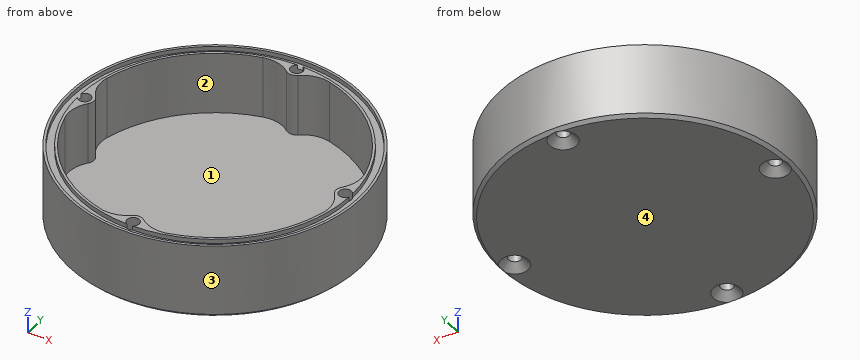
from build123d import *

# Parameters (mm, degrees)
F0_R      = 23.5
F1_DEPTH  = 12
F2_T      = -2
F3_SIZE   = 0.5
F4_R      = 1.5
F5_DEPTH  = 10
F6_R      = 5
F7_R      = 1
F8_DEPTH  = 12.001
F9_R      = 23.1
F9_R_2    = 21.9
F10_DEPTH = 0.7


# Not quite as in the source:
# - a fillet or chamfer that OpenCascade refuses, or shapes differently, is made with other operations: its cross-section is extruded or revolved along the edge and cut away or added


with BuildPart() as f1:
    # F0 (on Top) → F1 (new body)
    with BuildSketch(Plane.XY):
        Circle(F0_R)
    extrude(amount=F1_DEPTH)

    # F2
    f2_openings = [f1.faces().sort_by_distance(p)[0] for p in [
        (0, 0, 12),
    ]]
    offset(amount=F2_T, openings=f2_openings)

    # F3
    f3_edges = [f1.edges().sort_by_distance(p)[0] for p in [
        (-23.5, 0, 0),
    ]]
    chamfer(f3_edges, length=F3_SIZE)

    # F4 (on face) → F5 (join, through all)
    with BuildSketch(Plane.XY.offset(2)):
        with Locations((0, -21)):
            Circle(F4_R)
        with Locations((21, 0)):
            Circle(F4_R)
        with Locations((0, 21)):
            Circle(F4_R)
        with Locations((-21, 0)):
            Circle(F4_R)
    extrude(amount=F5_DEPTH)

    # F6
    f6_edges = [f1.edges().sort_by_distance(p)[0] for p in [
        (-21.452381, 1.430158, 7),
        (-21.452381, -1.430158, 7),
        (-1.430158, 21.452381, 7),
        (1.430158, 21.452381, 7),
        (21.452381, -1.430158, 7),
        (21.452381, 1.430158, 7),
        (-1.430158, -21.452381, 7),
        (1.430158, -21.452381, 7),
    ]]
    fillet(f6_edges, radius=F6_R)

    # F7 (on face) → F8 (cut, through all)
    with BuildSketch(Plane.XY.offset(12)):
        with Locations((0, -21)):
            Circle(F7_R)
        with Locations((21, 0)):
            Circle(F7_R)
        with Locations((0, 21)):
            Circle(F7_R)
        with Locations((-21, 0)):
            Circle(F7_R)
    extrude(amount=-F8_DEPTH, mode=Mode.SUBTRACT)

    # F9 (on face) → F10 (cut)
    with BuildSketch(Plane.XY.offset(12)):
        Circle(F9_R)
        Circle(F9_R_2, mode=Mode.SUBTRACT)
    extrude(amount=-F10_DEPTH, mode=Mode.SUBTRACT)

    # F11: chamfer of 1.2 on 4 edges, made by hand

    # F11_s1 → F11_t2 (revolve, cut)
    with BuildSketch(Plane.XZ.offset(-21)):
        Polygon((2.2, 0), (1, 1.2), (1, 0), align=None)
    revolve(axis=Axis((0, 21, 0), (0, 0, 1)), mode=Mode.SUBTRACT)

    # F11_s3 → F11_t4 (revolve, cut)
    with BuildSketch(Plane.XZ):
        Polygon((23.2, 0), (22, 1.2), (22, 0), align=None)
    revolve(axis=Axis((21, 0, 0), (0, 0, 1)), mode=Mode.SUBTRACT)

    # F11_s5 → F11_t6 (revolve, cut)
    with BuildSketch(Plane.XZ.offset(21)):
        Polygon((2.2, 0), (1, 1.2), (1, 0), align=None)
    revolve(axis=Axis((0, -21, 0), (0, 0, 1)), mode=Mode.SUBTRACT)

    # F11_s7 → F11_t8 (revolve, cut)
    with BuildSketch(Plane.XZ):
        Polygon((-18.8, 0), (-20, 1.2), (-20, 0), align=None)
    revolve(axis=Axis((-21, 0, 0), (0, 0, 1)), mode=Mode.SUBTRACT)


solid = f1.part
CAD build for the part. Positions are in the model's coordinates, mm. Face numbers are marked on the shaded views. Give positions to 0.01 mm unless a question says otherwise; leave off trailing zeros. Answer in a Markdown table with one row per item. Add a question column.
Item 1: Mould opens along Y. For the marked faces 1, 2, 3 and 4 say: +Y half, -Y half, draft (parallel to the pull), parting line (faces both ways), or undercut.
Item 2: Probe probe 1 along Y at (x, z) = (0, 11.8); probe 2 along Y at (x, z) = (0, 6); probe 3 along Z at (x, y) = (9.5, -6). List the from-to ranges inside material, lowest first.
Item 3: Drop flat-ended pins along their axis: P1, Ø6, axis at y = 16.5, z = 9.5, coming from the -X side; P2, Ø6, axis at x = 6.5, z = 4.5, coming from the +Y side; P3, Ø2.5, axis at x = 0, y = -21, coming from the +Z side; P4, Ø1, axis at x = -4, z = 6, coming from the -Y side. Give the stop position or say it passes through.
Reply:
| question | item | result |
|---|---|---|
| 1 | face 1 | undercut |
| 1 | face 2 | undercut |
| 1 | face 3 | parting line |
| 1 | face 4 | draft |
| 2 | probe 1 | y = -23.5 to -23.1, -20 to -19.5, 19.5 to 20, 23.1 to 23.5 |
| 2 | probe 2 | y = -23.5 to -22, -20 to -19.5, 19.5 to 20, 22 to 23.5 |
| 2 | probe 3 | z = 0 to 2 |
| 3 | P1 | stops at x = -19.24 |
| 3 | P2 | stops at y = 23.24 |
| 3 | P3 | stops at z = 12 |
| 3 | P4 | stops at y = -23.24 |
